Build history of the part. All positions in model axes, mm. A direction names the side the tool comes from. Give positions to 0.01 mm unless a question says otherwise; leave off trailing zeros. Loops run counter-clockwise (first coordinate to the right, second up) from the corner with the lowest first, then second, coordinate; pieces in that order, holes last. Notation, with made-up numbers: (-40, 73.25) -> (-5, 73.25) arc R27 ccw to (-5, 108.25) -> close; hole circle Ø5 at (50, 81.25). An arc over 180 degrees is marked (long way). Answer as a JSON object with one key per item and string values. Group by question number.
Q1. Band-saw the part on A-A, the plane y = 23.57. Write the cut outline in (x, z), plus the area to 3 significant figures.
Q2. Wall check: probe 1 along Y at (x, z) = (-23.57, 8.75); probe 2 along Y at (x, z) = (0, 1.2) (3 decimals); probe 3 along Y at (x, z) = (10.25, 39.5). Give the ranges that are in metal, low to high. Write a range as from..to.
Q3. Band-saw the part on D-D, the plane x = 0. Count the separate pieces of the cut face and the enclosed holes in it, plus the area to 3 significant figures.
Q4. Two-plate mould, pull along Z, no slides. Class faces 1 (the flat face through (-8, -13, 3)), 2 (the flat face through (-18, -10, 38)), 3 (the cylindrical face through (0.05, -18.8, 38.83)), 4 (the cylindrical face through (25.1, 24.1, 5.6)): pulls with the +Z half, pulls with the -Z half, needs draft (parallel to the pull), parting line crosses it, or undercut.
Q5. Drop flat-ended pins along their axis: pin 1 (4.5 mm diameter, centred on x = 17.75, y = 10.25, fed in from -Z); pin 2 (5 mm diameter, centred on y = 14, z = 24.5, fed in from +X); pin 3 (5 mm diameter, centred on y = 0.5, z = 31.5, fed in from -X); pin 4 (1.8 mm diameter, centred on x = -10, y = 18.5, fed in from +Z). Give the stop position or say it passes through.
Q6. Tool access for faces 5 (the flat face through (-22, 0, 26)), 6 (the cylindrical face through (-24.856, 22.584, 5.615)), 7 (the cylindrical face through (-9.442, 16.201, 39.774)), 8 (the flat face through (22, 0, 26)), 9 (the cylindrical face through (-27.3, 27.34, 5.42)): list every direction of +Z, -Z, +X, -X, +Y, -Y with a clear straight run to the whole face (end or side of a thin tool).
Q7. Band-saw the part on C-C, the plane z = 32.5. Write the cut outline in (x, y), plus the area to 3 significant figures.
from build123d import *

# Parameters (mm, degrees)
BOSS_EXTRUDE1_DEPTH  = 11
BOSS_EXTRUDE2_DEPTH  = 41.5
SKETCH4_R            = 1.75
CUT_EXTRUDE1_DEPTH   = 3.5
LPATTERN1_COUNT      = 2
LPATTERN1_PITCH      = 28.991378029
LPATTERN1_COUNT_DIR2 = 2
LPATTERN1_PITCH_DIR2 = 28.991378029
LPATTERN2_COUNT      = 2
LPATTERN2_PITCH      = 47.14
LPATTERN2_COUNT_DIR2 = 2
LPATTERN2_PITCH_DIR2 = 47.14


with BuildPart() as part:
    # Sketch1 → Boss-Extrude1 (new body)
    with BuildSketch(Plane.XY):
        with BuildLine():
            Line((-25.2, -28.2), (25.2, -28.2))
            ThreePointArc((25.2, -28.2), (27.321320344, -27.321320344), (28.2, -25.2))
            Line((28.2, -25.2), (28.2, 25.2))
            ThreePointArc((28.2, 25.2), (27.321320344, 27.321320344), (25.2, 28.2))
            Line((25.2, 28.2), (-25.2, 28.2))
            ThreePointArc((-25.2, 28.2), (-27.321320344, 27.321320344), (-28.2, 25.2))
            Line((-28.2, 25.2), (-28.2, -25.2))
            ThreePointArc((-28.2, -25.2), (-27.321320344, -27.321320344), (-25.2, -28.2))
        make_face()
    extrude(amount=BOSS_EXTRUDE1_DEPTH)

    # Sketch2 → Boss-Extrude2 (add)
    with BuildSketch(Plane.XY):
        with BuildLine():
            Line((-21, -22), (21, -22))
            ThreePointArc((21, -22), (21.707106781, -21.707106781), (22, -21))
            Line((22, -21), (22, 21))
            ThreePointArc((22, 21), (21.707106781, 21.707106781), (21, 22))
            Line((21, 22), (-21, 22))
            ThreePointArc((-21, 22), (-21.707106781, 21.707106781), (-22, 21))
            Line((-22, 21), (-22, -21))
            ThreePointArc((-22, -21), (-21.707106781, -21.707106781), (-21, -22))
        make_face()
    extrude(amount=BOSS_EXTRUDE2_DEPTH)

    # Sketch3 → Cut-Revolve1 (revolve, cut)
    with BuildSketch(Plane(origin=(0, 0, 0), x_dir=(0, 0, -1), z_dir=(1, 0, 0)), mode=Mode.PRIVATE) as cut_revolve1_sk:
        Polygon((-41.5, 0), (-41.5, 16.288675135), (-41, 16), (-33.5, 16), (-33.5, 15), (-3, 15), (-3, 19.065), (-0.5, 19.065), (0, 19.565), (0, 0), align=None)
    revolve(cut_revolve1_sk.sketch.rotate(Axis((0, 0, 0), (0, 0, 1)), 270), axis=Axis((0, 0, 0), (0, 0, 1)), mode=Mode.SUBTRACT)

    # Sketch4 → Cut-Extrude1 (cut)
    with BuildSketch(Plane.XY.offset(41.5)):
        with Locations((17.753520778, 10.25)):
            Circle(SKETCH4_R)
    cut_extrude1 = extrude(amount=-CUT_EXTRUDE1_DEPTH, mode=Mode.SUBTRACT)

    # LPattern1: Cut-Extrude1 2 × 2
    with Locations(*[Vector(-0.9659258262890682, 0.2588190451025211, 0) * (i * LPATTERN1_PITCH) + Vector(-0.2588190451025205, -0.9659258262890683, 0) * (j * LPATTERN1_PITCH_DIR2) for i in range(LPATTERN1_COUNT) for j in range(LPATTERN1_COUNT_DIR2) if (i, j) != (0, 0)]):
        add(cut_extrude1, mode=Mode.SUBTRACT)

    # Sketch6 → Cut-Revolve2 (revolve, cut)
    with BuildSketch(Plane(origin=(23.57, 0, 0), x_dir=(0, 0, -1), z_dir=(1, 0, 0)), mode=Mode.PRIVATE) as cut_revolve2_sk:
        Polygon((-11.935884786, 23.57), (-11, 25.191), (-0.379, 25.191), (0, 25.57), (0, 23.57), align=None)
    cut_revolve2 = revolve(cut_revolve2_sk.sketch.rotate(Axis((23.57, 23.57, 0), (0, 0, 1)), 270), axis=Axis((23.57, 23.57, 0), (0, 0, 1)), mode=Mode.SUBTRACT)

    # LPattern2: Cut-Revolve2 2 × 2
    with Locations(*[(-i * LPATTERN2_PITCH, -j * LPATTERN2_PITCH_DIR2, 0) for i in range(LPATTERN2_COUNT) for j in range(LPATTERN2_COUNT_DIR2) if (i, j) != (0, 0)]):
        add(cut_revolve2, mode=Mode.SUBTRACT)

    # Sketch8 → Cut-Revolve3 (revolve, cut)
    with BuildSketch(Plane.XY.offset(37.6), mode=Mode.PRIVATE) as cut_revolve3_sk:
        Polygon((-22, 0), (-22, 1.5), (-21.7295, 1.2295), (-15.8, 1.2295), (-15.8, 0), align=None)
    revolve(cut_revolve3_sk.sketch.rotate(Axis((-15.8, 0, 37.6), (-1, 0, 0)), 270), axis=Axis((-15.8, 0, 37.6), (-1, 0, 0)), mode=Mode.SUBTRACT)

    # Sketch9 → Cut-Revolve4 (revolve, cut)
    with BuildSketch(Plane.XY.offset(37.6), mode=Mode.PRIVATE) as cut_revolve4_sk:
        Polygon((0, -22), (-1.5, -22), (-1.2295, -21.7295), (-1.2295, -15.8), (0, -15.8), align=None)
    revolve(cut_revolve4_sk.sketch.rotate(Axis((0, -15.8, 37.6), (0, -1, 0)), 90), axis=Axis((0, -15.8, 37.6), (0, -1, 0)), mode=Mode.SUBTRACT)

    # Sketch10 → Cut-Revolve5 (revolve, cut)
    with BuildSketch(Plane.XY.offset(37.6), mode=Mode.PRIVATE) as cut_revolve5_sk:
        Polygon((22, 0), (22, -1.5), (21.7295, -1.2295), (15.8, -1.2295), (15.8, 0), align=None)
    revolve(cut_revolve5_sk.sketch.rotate(Axis((15.8, 0, 37.6), (1, 0, 0)), 90), axis=Axis((15.8, 0, 37.6), (1, 0, 0)), mode=Mode.SUBTRACT)

    # Sketch11 → Cut-Revolve6 (revolve, cut)
    with BuildSketch(Plane.XY.offset(37.6), mode=Mode.PRIVATE) as cut_revolve6_sk:
        Polygon((0, 22), (1.5, 22), (1.2295, 21.7295), (1.2295, 15.8), (0, 15.8), align=None)
    revolve(cut_revolve6_sk.sketch.rotate(Axis((0, 15.8, 37.6), (0, 1, 0)), 270), axis=Axis((0, 15.8, 37.6), (0, 1, 0)), mode=Mode.SUBTRACT)


solid = part.part
Worked answers:
{
 "1": {"outline": "(-28.2, 0) -> (-25.57, 0) -> (-25.19, 0.38) -> (-25.19, 11) -> (-28.2, 11) -> close; (-21.95, 0.38) -> (-21.57, 0) -> (21.57, 0) -> (21.95, 0.38) -> (21.95, 11) -> (-21.95, 11) -> close; (25.19, 0.38) -> (25.57, 0) -> (28.2, 0) -> (28.2, 11) -> (25.19, 11) -> close", "area": "549 mm2"},
 "2": {"probe 1": "-28.2..-25.19, -21.95..21.95, 25.19..28.2", "probe 2": "-28.2..-19.065, 19.065..28.2", "probe 3": "-22..-19.5, -16..-12.29, 12.29..22"},
 "3": {"separate pieces": "4", "enclosed holes": "0", "area": "647 mm2"},
 "4": {"face 1": "pulls with the -Z half", "face 2": "pulls with the +Z half", "face 3": "undercut", "face 4": "needs draft"},
 "5": {"pin 1": "z = 0", "pin 2": "x = 22", "pin 3": "x = -22", "pin 4": "z = 38"},
 "6": {"face 5": "+Z, -X, +Y, -Y", "face 6": "+Z, -Z", "face 7": "+Z", "face 8": "+Z, +X, +Y, -Y", "face 9": "+Z, -Z, -X, +Y"},
 "7": {"outline": "(-22, -21) arc R1 ccw to (-21, -22) -> (21, -22) arc R1 ccw to (22, -21) -> (22, 21) arc R1 ccw to (21, 22) -> (-21, 22) arc R1 ccw to (-22, 21) -> close; hole circle Ø30 at (0, 0)", "area": "1,230 mm2"}
}
